Read the model definition and answer for the solid it produces. Units are mm, in the model's axes. A direction names the side the tool comes from. Round coordinates to 2 decimals unless told otherwise and drop trailing zeros. Order: outer loops, then holes, each group sorted by start corner. A loop starts at its lowest first (then second) coordinate and runs counter-clockwise, first axis right, second up.
from build123d import *

# Parameters (mm, degrees)
F0_W      = 50.8
F0_H      = 38.1
F1_DEPTH  = 25.4
F2_W      = 12.7
F2_H      = 19.05
F3_DEPTH  = 19.05
F4_W      = 12.7
F4_H      = 25.4
F5_DEPTH  = 19.05
F6_W      = 12.7
F6_H      = 6.35
F7_DEPTH  = 19.05
F9_DEPTH  = 25.4
F11_DEPTH = 25.4


with BuildPart() as f1:
    # F0 (on Front) → F1 (new body)
    with BuildSketch(Plane.XZ):
        with Locations((25.4, 19.05)):
            Rectangle(F0_W, F0_H)
    extrude(amount=F1_DEPTH)

    # F2 (on face) → F3 (cut)
    with BuildSketch(Plane(origin=(0, 0, 0), x_dir=(0, -1, 0), z_dir=(-1, 0, 0))):
        with Locations((19.05, 28.575)):
            Rectangle(F2_W, F2_H)
    extrude(amount=-F3_DEPTH, mode=Mode.SUBTRACT)

    # F4 (on face) → F5 (cut)
    with BuildSketch(Plane.YZ.offset(50.8)):
        with Locations((-19.05, 25.4)):
            Rectangle(F4_W, F4_H)
    extrude(amount=-F5_DEPTH, mode=Mode.SUBTRACT)

    # F6 (on face) → F7 (cut)
    with BuildSketch(Plane(origin=(0, 0, 0), x_dir=(0, -1, 0), z_dir=(-1, 0, 0))):
        with Locations((19.05, 15.875)):
            Rectangle(F6_W, F6_H)
    extrude(amount=-F7_DEPTH, mode=Mode.SUBTRACT)

    # F8 (on face) → F9 (cut)
    with BuildSketch(Plane(origin=(19.05, 0, 0), x_dir=(0, -1, 0), z_dir=(-1, 0, 0))):
        Polygon((25.4, 38.1), (12.7, 38.1), (25.4, 12.7), align=None)
    extrude(amount=-F9_DEPTH, mode=Mode.SUBTRACT)

    # F10 (on face) → F11 (cut)
    with BuildSketch(Plane(origin=(0, 0, 0), x_dir=(-1, 0, 0), z_dir=(0, 1, 0))):
        Polygon((-50.8, 12.7), (-38.1, 38.1), (-50.8, 38.1), align=None)
    extrude(amount=-F11_DEPTH, mode=Mode.SUBTRACT)


solid = f1.part
Q1. A cutting plane is placed at B-B, the plane y = -20.75. Give the vertices of the cut face in (x, z), plus the area to 3 significant figures.
Outcome:
outline: (0, 0) - (50.8, 0) - (50.8, 12.7) - (31.75, 12.7) - (31.75, 22) - (19.05, 22) - (19.05, 12.7) - (0, 12.7) - close
area: 763 mm2
Q2. A cutting plane is placed at D-D, the plane y = -4.75. Give the vertices of the cut face in (x, z), plus the area to 3 significant figures.
Outcome:
outline: (0, 0) - (50.8, 0) - (50.8, 12.7) - (38.1, 38.1) - (0, 38.1) - close
area: 1,770 mm2
Q3. A cutting plane is placed at C-C, the plane x = 42. Give the vertices of the cut face in (y, z), plus the area to 3 significant figures.
Outcome:
outline: (-25.4, 0) - (0, 0) - (0, 30.3) - (-12.7, 30.3) - (-12.7, 12.7) - (-25.4, 12.7) - close
area: 546 mm2
Q4. For faces 1 (the face through (39, -12.7, 22)), 2 (the face through (25, -13, 0)), 3 (the face through (19.05, -16, 20)), determine the directions among +Z, -Z, +X, -X, +Y, -Y from which every point of the face is accessible in a straight line to the end or side of a thin tool.
Outcome:
face 1: +Z, +X, -Y
face 2: -Z, +X, -X, +Y, -Y
face 3: +Z, -X, -Y
Q5. Straight lines are drawn through the part: probe 1 along X at (y, z) = (-14, 34.5); probe 2 along Z at (x, y) = (41, -16.25); probe 3 along Y at (x, z) = (14, 17). For each, find the intervals that lie inside material, in ascending order.
Outcome:
probe 1: x = 19.05 to 31.75
probe 2: z = 0 to 12.7
probe 3: y = -12.7 to 0
Q6. Flat-ended cylindrical pins translate along their axes: pin 1 (2 mm diameter, centred on y = -3, z = 23.5, fed in from +X); pin 2 (9.5 mm diameter, centred on x = 44.5, z = 30.5, fed in from -Y); pin 3 (2 mm diameter, centred on y = -7, z = 20.5, fed in from +X); pin 4 (2 mm diameter, centred on y = -5.5, z = 9.5, fed in from -X). Find the tip coordinate at first contact, or state that the pin passes through.
Outcome:
pin 1: stops at x = 45.9
pin 2: stops at y = -12.7
pin 3: stops at x = 47.4
pin 4: stops at x = 0
Q7. A cutting plane is placed at A-A, the plane z = 33.5. Give the vertices of the cut face in (x, y).
Outcome:
outline: (0, -12.7) - (19.05, -12.7) - (19.05, -15) - (31.75, -15) - (31.75, -12.7) - (40.4, -12.7) - (40.4, 0) - (0, 0) - close
